Could you check a few things on this model? Use its own coordinates, in mm. A direction names the side the tool comes from. Coordinates: 2 decimals unless noted, no trailing zeros.
```python
from build123d import *

# Parameters (mm, degrees)
F0_W     = 21
F0_H     = 17
F0_H_2   = 15
F0_H_3   = 13
F0_H_4   = 12
F1_DEPTH = 40
F2_R     = 2


with BuildPart() as f1:
    # F0 (on Front) → F1 (new body)
    with BuildSketch(Plane.XZ):
        with BuildLine():
            Line((-187.7269284463, 10), (-187.7269284463, 0))
            Line((-187.7269284463, 0), (-177.7269284463, 0))
            Line((-177.7269284463, 0), (-156.7269284463, 0))
            Line((-156.7269284463, 0), (-146.7269284463, 0))
            Line((-146.7269284463, 0), (-125.7269284463, 0))
            Line((-125.7269284463, 0), (-115.7269284463, 0))
            Line((-115.7269284463, 0), (-94.7269284463, 0))
            Line((-94.7269284463, 0), (-84.7269284463, 0))
            Line((-84.7269284463, 0), (-63.7269284463, 0))
            Line((-63.7269284463, 0), (-51.7269284463, 0))
            Line((-51.7269284463, 0), (-37.7269284463, 0))
            Line((-37.7269284463, 0), (-37.7269284463, 33))
            add(Edge.make_bspline(
                [(-178.7269284463, 50), (-171.8501135131, 45.8291458601), (-155.9934821594, 36.5832092462), (-116.9716909033, 31.7407768444), (-52.5012909301, 26.3666718297), (-41.333494482, 31.3189487613), (-37.7269284463, 33)],
                knots=[0, 0, 0, 0, 0.2135053975, 0.491145081, 0.8357316178, 1, 1, 1, 1], degree=3))
            Line((-178.7269284463, 50), (-187.7269284463, 50))
            Line((-187.7269284463, 50), (-187.7269284463, 10))
        make_face()
        with Locations((-167.2269284463, 18.5)):
            Rectangle(F0_W, F0_H, mode=Mode.SUBTRACT)
        with Locations((-136.2269284463, 17.5)):
            Rectangle(F0_W, F0_H_2, mode=Mode.SUBTRACT)
        with Locations((-105.2269284463, 16.5)):
            Rectangle(F0_W, F0_H_3, mode=Mode.SUBTRACT)
        with Locations((-74.2269284463, 16)):
            Rectangle(F0_W, F0_H_4, mode=Mode.SUBTRACT)
    extrude(amount=F1_DEPTH)

    # F2
    f2_edges = [f1.edges().sort_by_distance(p)[0] for p in [
        (-109.525437, -40, 31.392581),
        (-183.226928, -40, 50),
        (-187.726928, -40, 25),
        (-112.726928, -40, 0),
        (-37.726928, -40, 16.5),
        (-167.226928, -40, 10),
        (-177.726928, -40, 18.5),
        (-167.226928, -40, 27),
        (-156.726928, -40, 18.5),
        (-136.226928, -40, 10),
        (-146.726928, -40, 17.5),
        (-136.226928, -40, 25),
        (-125.726928, -40, 17.5),
        (-105.226928, -40, 10),
        (-115.726928, -40, 16.5),
        (-105.226928, -40, 23),
        (-94.726928, -40, 16.5),
        (-74.226928, -40, 10),
        (-84.726928, -40, 16),
        (-74.226928, -40, 22),
        (-63.726928, -40, 16),
        (-37.726928, -20, 33),
        (-178.726928, -20, 50),
        (-109.525437, 0, 31.392581),
        (-187.726928, -20, 50),
        (-187.726928, -20, 0),
        (-187.726928, 0, 25),
        (-183.226928, 0, 50),
        (-112.726928, 0, 0),
        (-37.726928, 0, 16.5),
        (-167.226928, 0, 10),
        (-177.726928, 0, 18.5),
        (-167.226928, 0, 27),
        (-156.726928, 0, 18.5),
        (-136.226928, 0, 10),
        (-146.726928, 0, 17.5),
        (-136.226928, 0, 25),
        (-125.726928, 0, 17.5),
        (-105.226928, 0, 10),
        (-115.726928, 0, 16.5),
        (-105.226928, 0, 23),
        (-94.726928, 0, 16.5),
        (-74.226928, 0, 10),
        (-84.726928, 0, 16),
        (-74.226928, 0, 22),
        (-63.726928, 0, 16),
        (-37.726928, -20, 0),
    ]]
    fillet(f2_edges, radius=F2_R)


solid = f1.part
```
1. On a 3-axis mill with a long thin cutter (end or side, diameter ignored), from which of +Z, -Z, +X, -X, +Y, -Y can I reach the whole of each face in a straight line? I mean faces 1 (the face through (-182, -20, 50)), 2 (the face through (-136, -20, 25)). Say none if no direction works.
Verdict:
face 1: +Z, +X, -X, +Y, -Y
face 2: +Y, -Y
2. I want a section at A-A on z = 20.5. Give the number of separate pieces and of enclosed holes in the cut face, plus the area to 3 significant figures.
Verdict:
separate pieces: 5
enclosed holes: 0
area: 2,620 mm2
3. Please list where these lines run through material, in increasing order: line 1 along X through (y, z) = (-6, 22.5); line 2 along X through (y, z) = (-12, 19.5); line 3 along X through (y, z) = (-15, 26.5).
Verdict:
line 1: x = -187.73 to -177.73, -156.73 to -146.73, -125.73 to -115.73, -94.73 to -37.73
line 2: x = -187.73 to -177.73, -156.73 to -146.73, -125.73 to -115.73, -94.73 to -84.73, -63.73 to -37.73
line 3: x = -187.73 to -177.73, -156.73 to -37.73
4. For pin 1 (3 mm diameter, centred on x = -153.5, z = 36.5, fed in from -Y); pin 2 (23 mm diameter, centred on x = -108, y = -18, fed in from +Z); pin 3 (12 mm diameter, centred on x = -167, y = -34.5, fed in from +Z); pin 4 (6 mm diameter, centred on y = -6, z = 34, fed in from +X), each with a flat end and sliding along its axis, tell me the tip position at first contact or that it passes through.
Verdict:
pin 1: stops at y = -40
pin 2: stops at z = 32.38
pin 3: stops at z = 46.6
pin 4: stops at x = -38.05
5. If we mould it in two halves opening along Z, with no side actions, what happens to faces 3 (the face through (-114, -20, 0)), 4 (the face through (-63.727, -20, 16)), 5 (the face through (-118, 0, 18))? For each: pulls with the +Z half, pulls with the -Z half, needs draft (parallel to the pull), parting line crosses it, or undercut.
Verdict:
face 3: pulls with the -Z half
face 4: undercut
face 5: needs draft
